from build123d import *

# Parameters (mm, degrees)
FILLET1_R           = 6
CUT_EXTRUDE8_DEPTH  = 10
SKETCH6_W           = 55
SKETCH6_H           = 16.343735742
CUT_EXTRUDE15_DEPTH = 20
SKETCH7_R           = 5.198582593
CUT_EXTRUDE16_DEPTH = 10
BOSS_EXTRUDE1_DEPTH = 60
SKETCH9_R           = 12
CUT_EXTRUDE17_DEPTH = 60


with BuildPart() as part:
    # Sketch1 → Revolve1 (revolve)
    with BuildSketch(Plane.XY, mode=Mode.PRIVATE) as revolve1_sk:
        Polygon((0, 0), (0, 14.656862745), (55, 14.656862745), (55, 0), (120, 0), (120, -24), (0, -24), align=None)
    revolve(revolve1_sk.sketch.rotate(Axis((-5.281550193, -24, 0), (1, 0, 0)), 90), axis=Axis((-5.281550193, -24, 0), (1, 0, 0)))

    # Fillet1
    fillet1_edges = [part.edges().sort_by_distance(p)[0] for p in [
        (120, -24, -24),
    ]]
    fillet(fillet1_edges, radius=FILLET1_R)

    # Sketch2 → Cut-Extrude8 (cut)
    with BuildSketch(Plane(origin=(0, 0, 0), x_dir=(1, 0, 0), z_dir=(0, 1, 0))):
        with BuildLine():
            Line((70.195378011, 8), (96.812319076, 8))
            ThreePointArc((96.812319076, 8), (104.812319076, 0), (96.812319076, -8))
            Line((96.812319076, -8), (70.195378011, -8))
            ThreePointArc((70.195378011, -8), (62.195378011, 0), (70.195378011, 8))
        make_face()
    extrude(amount=-CUT_EXTRUDE8_DEPTH, mode=Mode.SUBTRACT)

    # Sketch6 → Cut-Extrude15 (cut)
    with BuildSketch(Plane(origin=(0, 0, 0), x_dir=(1, 0, 0), z_dir=(0, 1, 0))):
        with Locations((27.5, 0.064856094)):
            Rectangle(SKETCH6_W, SKETCH6_H)
    extrude(amount=CUT_EXTRUDE15_DEPTH, mode=Mode.SUBTRACT)

    # Sketch7 → Cut-Extrude16 (cut)
    with BuildSketch(Plane(origin=(0, 0, 0), x_dir=(1, 0, 0), z_dir=(0, 1, 0))):
        with Locations(Location((27.964324109, 0, 0), (0, 0, 270))):
            Circle(SKETCH7_R)
    extrude(amount=-CUT_EXTRUDE16_DEPTH, mode=Mode.SUBTRACT)

    # Sketch8 → Boss-Extrude1 (add)
    with BuildSketch(Plane.ZY):
        with BuildLine():
            Line((10, -12.82210563), (10, -46.757053375))
            ThreePointArc((10, -46.757053375), (0, -56.757053375), (-10, -46.757053375))
            Line((-10, -46.757053375), (-10, -12.82210563))
            ThreePointArc((-10, -12.82210563), (0, -2.82210563), (10, -12.82210563))
        make_face()
    extrude(amount=BOSS_EXTRUDE1_DEPTH)

    # Sketch9 → Cut-Extrude17 (cut)
    with BuildSketch(Plane(origin=(0, 0, -10), x_dir=(-1, 0, 0), z_dir=(0, 0, -1))):
        with Locations(Location((31.933586772, -30.014179295, 0), (0, 0, 90))):
            Circle(SKETCH9_R)
    extrude(amount=-CUT_EXTRUDE17_DEPTH, mode=Mode.SUBTRACT)


solid = part.part
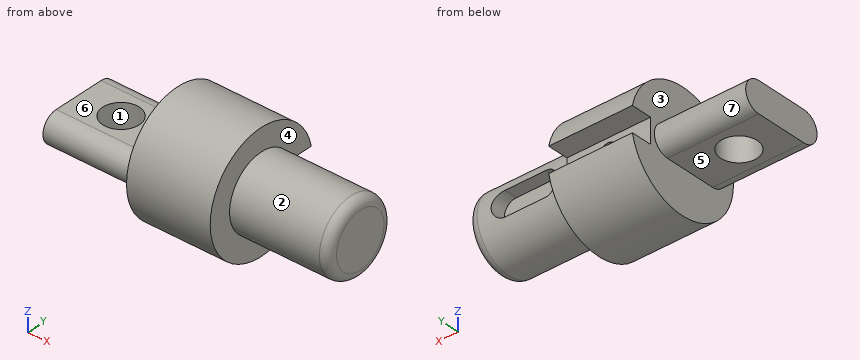
Work out the finished part from the listing and answer in its coordinate system (mm). Face numbers are marked on the shaded views. A direction names the side the tool comes from. Give positions to 0.01 mm unless a question says otherwise; leave off trailing zeros. Write each loop counter-clockwise with the first axis right and the second up, starting at its lowest first coordinate (ties: lowest second). Pieces come first, ordered by that corner, then holes. Notation, with made-up numbers: (4, 12) - (18, 12) arc R16 cw to (18, 34) - close; hole circle Ø9 at (36.5, 33). An arc over 180 degrees is marked (long way). One line per item, written item: value. Start each with the question number.
1. Find section B-B (y = -24). Write down the section's boundary in (x, z).
2. Find section C-C (y = 4). Write down the section's boundary in (x, z), then the cut area to 3 significant figures.
3. Given pin 1 (15 mm diameter, centred on x = 25, y = 6.5, fed in from +Z); pin 2 (4.5 mm diameter, centred on x = 79, y = -7, fed in from -Z); pin 3 (8.5 mm diameter, centred on x = 29.5, z = 1, fed in from +Y), each flat-ended and moving along its own axis, determine where each tip first touches the part or whether it passes through.
4. For a pull along Y with two mould halves and no side action, classify the marked faces 1, 2 and 3 as +Y half, -Y half, draft (parallel to the pull), parting line (faces both ways), or undercut.
5. For the marked faces 4, 5, 6 and 7, determine the directions among +Z, -Z, +X, -X, +Y, -Y from which every point of the face is accessible in a straight line to the end or side of a thin tool.
6. Find section D-D (x = 80). Write down the section's boundary in (y, z), then the cut area to 3 significant figures.
7. Find section A-A (x = -26). Write down the section's boundary in (y, z), then the cut area to 3 significant figures.
8. Consider probe 1 along X at (y, z) = (-22.5, -14); probe 2 along X at (y, z) = (-22.5, 28); probe 3 along X at (y, z) = (-36, -4.5). Determine where each line is inside the solid, lowest interval first.
Geometry results:
1. outline: (-60, -10) - (-42.32, -10) - (-42.32, 10) - (-60, 10) - close; (-21.55, -10) - (0, -10) - (0, -38.66) - (55, -38.66) - (55, -24) - (114, -24) arc R6 ccw to (120, -18) - (120, 18) arc R6 ccw to (114, 24) - (55, 24) - (55, 38.66) - (0, 38.66) - (0, 10) - (-21.55, 10) - close
2. outline: (0, -26.65) - (55, -26.65) - (55, -8.24) - (0, -8.24) - close; (0, 8.11) - (55, 8.11) - (55, 26.65) - (0, 26.65) - close
2. area: 2,030 mm2
3. pin 1: z = 31.07
3. pin 2: z = -18.93
3. pin 3: y = 0
4. face 1: undercut
4. face 2: parting line
4. face 3: draft
5. face 4: +X
5. face 5: -Z, -X, +Y, -Y
5. face 6: +Z, -X, +Y, -Y
5. face 7: -X, +Y
6. outline: (-10, -8) - (-10, 8) - (-1.37, 8) arc R24 ccw (long way) to (-1.37, -8) - close
6. area: 1,660 mm2
7. outline: (-46.76, -10) - (-40.44, -10) - (-40.44, 10) - (-46.76, 10) arc R10 ccw to start; (-19.58, -10) - (-12.82, -10) arc R10 ccw to (-12.82, 10) - (-19.58, 10) - close
7. area: 576 mm2
8. probe 1: 0 to 120
8. probe 2: 0 to 55
8. probe 3: -60 to -42.33, -21.53 to 120
